Autodesk Inventor part; units mm, degrees
ref_plane "YZ Plane" through (0, 0, 0) normal (1, 0, 0) x (0, 1, 0)
ref_plane "XZ Plane" through (0, 0, 0) normal (0, 1, 0) x (-1, 0, 0)
ref_plane "XY Plane" through (0, 0, 0) normal (0, 0, 1) x (1, 0, 0)
sketch "スケッチ1" plane through (0, 0, 0) normal (0, 0, 1) x (1, 0, 0)
  line L0 (-2, 8) -> (2, 8)
  line L1 (2, 8) -> (2, 0)
  line L2 (2, 0) -> (-2, 0)
  line L3 (-2, 0) -> (-2, 8)
  point P0 (0, 0)
  point P1 (0, 0)
  dimension "d0" = 8
  dimension "d1" = 4
extrude "押し出し1" add sketch "スケッチ1" along normal blind 25
sketch "スケッチ2" plane through (-2, 0, 0) normal (-1, 0, 0) x (0, 0, 1)
  line L0 (0, 0) -> (25, 6)
  line L1 (25, 0) -> (25, 8)
  line L2 (0, 8) -> (25, 8)
  line L3 (25, 8) -> (0, 8)
  line L4 (0, 8) -> (0, 0)
  line L5 (0, 8) -> (0, 0)
  line L6 (0, 0) -> (25, 0)
  line L7 (25, 8) -> (25, 0)
  line L8 (0, 8) -> (25, 8)
  point P0 (0, 0)
  dimension "d4" = 2
extrude "押し出し2" cut sketch "スケッチ2" against normal through all contours L0 L1 L6
sketch "スケッチ3" plane through (-2, 8, 0) normal (0, 1, 0) x (1, 0, 0)
  line L0 (4, 0) -> (4, -25)
  line L1 (4, 0) -> (2.75, -25)
  line L2 (2.75, -25) -> (1.25, -25)
  line L3 (1.25, -25) -> (0, 0)
  line L4 (4, 0) -> (0, 0)
  line L5 (4, -25) -> (0, -25)
  line L6 (4, 0) -> (0, 0)
  line L7 (0, 0) -> (0, -25)
  line L8 (4, -25) -> (0, -25)
  line L9 (4, 0) -> (4, -25)
  point P0 (2, 0)
  point P1 (2, -25)
  point P2 (2, 0)
  dimension "d7" = 1.5
extrude "押し出し3" cut sketch "スケッチ3" against normal through all contours L0 L5 L1 | L3 L5 L7
sketch "スケッチ4" plane through (0, 0, 0) normal (0, 0, -1) x (-1, 0, 0)
  circle A0 centre (0, 6) radius 0.8
  circle A1 centre (0, 2) radius 0.8
  line L0 (-2, 8) -> (2, 8)
  line L1 (2, 0) -> (-2, 0)
  point P0 (0, 0)
  point P1 (0, 8)
  dimension "d10" = 1.6
  dimension "d11" = 1.6
  dimension "d12" = 2
  dimension "d13" = 2
  dimension "d16" = 4
extrude "押し出し4" cut sketch "スケッチ4" against normal blind 5
properties part number "amtana"
Geometry: final body of the model. Coordinates: model frame, mm. A direction names the side the tool comes from. Coordinates: 2 decimals unless noted, no trailing zeros. Order: outer loops, then holes, each group sorted by start corner. A loop starts at its lowest first (then second) coordinate and runs counter-clockwise, first axis right, second up.
(1) Access query for faces 1 (the face through (1.523, 4.945, 9.547)), 2 (the face through (0, 6, 5)). Directions: +Z, -Z, +X, -X, +Y, -Y. A direction counts if a zero-diameter tool reaches every point of the face in a straight line with its end or side. Return the directions, or none.
(2) Draft query along Y for faces 3 (the face through (-0.03, 2.29, 9.55)), 4 (the face through (0, 2, 5)), 5 (the face through (0, 7, 25)). Return one class per face: pulls with the +Y half, pulls with the -Y half, needs draft (parallel to the pull), parting line crosses it, or undercut.
(3) Section query B-B (x = -1.15). Return the cut outline in (y, z).
(4) Section query A-A (y = 2). Return the cut outline in (x, z), plus the area to 3 significant figures.
(5) First-contact query: pin 1 (3 mm diameter, centred on y = 5, z = 19.5, fed in from +X); pin 2 (2 mm diameter, centred on x = -1, z = 7.5, fed in from -Y). Flat tips, straight axial feed; report the tip coordinate or a pass-through.
(6) Material intervals for probe 1 along Y at (x, z) = (0, 1.5); probe 2 along Y at (x, z) = (0, 2.65); probe 3 along Z at (x, y) = (-0.1, 6.5), sorted ascending.
(7) Section query C-C (z = 21). Return the cut outline in (x, y).
Solution:
1. face 1: +Z, +X, +Y, -Y
1. face 2: -Z
2. face 3: pulls with the -Y half
2. face 4: undercut
2. face 5: needs draft
3. outline: (0, 0) - (8, 0) - (8, 17) - (4.08, 17) - close
4. outline: (-2, 0) - (-0.8, 0) - (-0.8, 5) - (0.8, 5) - (0.8, 0) - (2, 0) - (1.58, 8.33) - (-1.58, 8.33) - close
4. area: 21.9 mm2
5. pin 1: stops at x = 1.1
5. pin 2: stops at y = 1.56
6. probe 1: y = 0.36 to 1.2, 2.8 to 5.2, 6.8 to 8
6. probe 2: y = 0.64 to 1.2, 2.8 to 5.2, 6.8 to 8
6. probe 3: z = 5 to 25
7. outline: (-0.95, 5.04) - (0.95, 5.04) - (0.95, 8) - (-0.95, 8) - close
